Work out the finished part from the listing and answer in its coordinate system (mm). A direction names the side the tool comes from. Give positions to 0.01 mm unless a question says otherwise; leave off trailing zeros. Loops run counter-clockwise (first coordinate to the right, second up) from the corner with the lowest first, then second, coordinate; pieces in that order, holes last. Notation, with made-up numbers: M -2.75,29.5 L 56.25,29.5 A8 cw 56.25,40.5 Z; hole C 65,-34.5 d2. An arc over 180 degrees is marked long. Answer as a JSON object with one key per item and string values. Group by question number.
```python
from build123d import *

# Parameters (mm, degrees)
BOSS_EXTRUDE1_DEPTH = 3


with BuildPart() as part:
    # Sketch1 → Boss-Extrude1 (new body)
    with BuildSketch(Plane(origin=(0, 0, 0), x_dir=(1, 0, 0), z_dir=(0, 1, 0))):
        Polygon((0, 52), (0, -57), (-76, -57), (-76, -37), (-73, -37), (-73, -12), (-76, -12), (-76, 12), (-73, 12), (-73, 37), (-76, 37), (-76, 52), (-45.6, 52), (-45.6, 57), (-15.2, 57), (-15.2, 52), align=None)
    boss_extrude1 = extrude(amount=BOSS_EXTRUDE1_DEPTH)

    # Mirror1: Boss-Extrude1 across plane
    add(boss_extrude1.mirror(Plane(origin=(0, 3, -52), x_dir=(0, 0, 1), z_dir=(-1, 0, 0))))


solid = part.part
```
Item 1: Find the intervals of material crossed by probe 1 along Z at (x, y) = (-9, 0.5); probe 2 along X at (y, z) = (1.9, -23.5), in increasing order. Write a range as [from, to].
Item 2: A cutting plane is placed at B-B (x = -61). Determine the outline of the cut face in (y, z).
Item 3: A tool of negligible diameter and unlimited length cuts with its end or side. For faces 1 (the flat face through (-76, 1, -44)), 2 (the flat face through (-74, 1, 12)), 3 (the flat face through (15.2, 1, -55)), 4 (the flat face through (-31, 1, -57)), 5 (the flat face through (73, 1, -24)), from which of +Z, -Z, +X, -X, +Y, -Y can it reach the whole face along a straight path? Write none if from no direction.
Item 4: A cutting plane is placed at A-A (y = 2.05). Determine the outline of the cut face in (x, z), and give its area (3 significant figures).
Item 5: A cutting plane is placed at C-C (z = -32). Determine the outline of the cut face in (x, y).
Item 6: Given pin 1 Ø0.9 at (y, z) = (1.5, 18.5) entering from +X; pin 2 Ø0.9 at (y, z) = (1, -54.5) entering from -X; pin 3 Ø0.9 at (x, y) = (54, 1.5) entering from -Z, each flat-ended and moving along its own axis, determine where each tip first touches the part or whether it passes through.
Item 7: For a pull along Z with two mould halves and no side action, classify faces 6 (the flat face through (-61, 1, -52)), 7 (the flat face through (45.6, 1, -54)), 8 (the flat face through (73, 1, 25)) as pulls with the +Z half, pulls with the -Z half, needs draft (parallel to the pull), parting line crosses it, or undercut.
The answers:
{
 "1": {"probe 1": "z = [-52, 57]", "probe 2": "x = [-73, 73]"},
 "2": {"outline": "M 0,-52 L 3,-52 L 3,57 L 0,57 Z"},
 "3": {"face 1": "+Z, -Z, -X, +Y, -Y", "face 2": "-X, +Y, -Y", "face 3": "-Z, +Y, -Y", "face 4": "-Z, +X, -X, +Y, -Y", "face 5": "+X, +Y, -Y"},
 "4": {"outline": "M -76,-52 L -45.6,-52 L -45.6,-57 L -15.2,-57 L -15.2,-52 L 15.2,-52 L 15.2,-57 L 45.6,-57 L 45.6,-52 L 76,-52 L 76,-37 L 73,-37 L 73,-12 L 76,-12 L 76,12 L 73,12 L 73,37 L 76,37 L 76,57 L -76,57 L -76,37 L -73,37 L -73,12 L -76,12 L -76,-12 L -73,-12 L -73,-37 L -76,-37 Z", "area": "16,600 mm^2"},
 "5": {"outline": "M -73,0 L 73,0 L 73,3 L -73,3 Z"},
 "6": {"pin 1": "stops at x = 73", "pin 2": "stops at x = -45.6", "pin 3": "stops at z = -52"},
 "7": {"face 6": "pulls with the -Z half", "face 7": "needs draft", "face 8": "undercut"}
}
